from build123d import *

# Parameters (mm, degrees)
BOSS_EXTRUDE1_DEPTH = 4
FILLET1_R           = 1
SKETCH2_W           = 6.5
SKETCH2_H           = 21
SKETCH2_W_2         = 3
SKETCH2_H_2         = 16
BOSS_EXTRUDE2_DEPTH = 3
CUT_EXTRUDE3_DEPTH  = 94.63893421


with BuildPart() as part:
    # Sketch1 → Boss-Extrude1 (new body)
    with BuildSketch(Plane.XY):
        Polygon((0, 0), (52, 0), (52, 4), (90.5, 4), (90.5, 19), (52, 19), (52, 23), (0, 23), align=None)
    extrude(amount=BOSS_EXTRUDE1_DEPTH)

    # Fillet1
    fillet1_edges = [part.edges().sort_by_distance(p)[0] for p in [
        (0, 23, 2),
        (52, 23, 2),
        (52, 19, 2),
        (90.5, 19, 2),
        (90.5, 4, 2),
        (52, 4, 2),
        (52, 0, 2),
        (0, 0, 2),
    ]]
    fillet(fillet1_edges, radius=FILLET1_R)

    # Sketch2 → Boss-Extrude2 (add)
    with BuildSketch(Plane.XY.offset(4)):
        with Locations((46.75, 11.5)):
            Rectangle(SKETCH2_W, SKETCH2_H)
        with Locations((46.75, 11.5)):
            Rectangle(SKETCH2_W_2, SKETCH2_H_2, mode=Mode.SUBTRACT)
    extrude(amount=BOSS_EXTRUDE2_DEPTH)

    # Sketch3 → Cut-Extrude3 (cut, through all)
    with BuildSketch(Plane(origin=(0, 0, 0), x_dir=(-1, 0, 0), z_dir=(0, 0, -1))):
        with BuildLine():
            Line((-53.7, 14), (-52.3, 14))
            ThreePointArc((-52.3, 14), (-51.734314575, 14.234314575), (-51.5, 14.8))
            Line((-51.5, 14.8), (-51.5, 16.2))
            ThreePointArc((-51.5, 16.2), (-51.734314575, 16.765685425), (-52.3, 17))
            Line((-52.3, 17), (-53.7, 17))
            ThreePointArc((-53.7, 17), (-54.265685425, 16.765685425), (-54.5, 16.2))
            Line((-54.5, 16.2), (-54.5, 14.8))
            ThreePointArc((-54.5, 14.8), (-54.265685425, 14.234314575), (-53.7, 14))
        make_face()
        with BuildLine():
            Line((-52.3, 10), (-53.7, 10))
            ThreePointArc((-53.7, 10), (-54.265685425, 10.234314575), (-54.5, 10.8))
            Line((-54.5, 10.8), (-54.5, 12.2))
            ThreePointArc((-54.5, 12.2), (-54.265685425, 12.765685425), (-53.7, 13))
            Line((-53.7, 13), (-52.3, 13))
            ThreePointArc((-52.3, 13), (-51.734314575, 12.765685425), (-51.5, 12.2))
            Line((-51.5, 12.2), (-51.5, 10.8))
            ThreePointArc((-51.5, 10.8), (-51.734314575, 10.234314575), (-52.3, 10))
        make_face()
        with BuildLine():
            Line((-53.7, 6), (-52.3, 6))
            ThreePointArc((-52.3, 6), (-51.734314575, 6.234314575), (-51.5, 6.8))
            Line((-51.5, 6.8), (-51.5, 8.2))
            ThreePointArc((-51.5, 8.2), (-51.734314575, 8.765685425), (-52.3, 9))
            Line((-52.3, 9), (-53.7, 9))
            ThreePointArc((-53.7, 9), (-54.265685425, 8.765685425), (-54.5, 8.2))
            Line((-54.5, 8.2), (-54.5, 6.8))
            ThreePointArc((-54.5, 6.8), (-54.265685425, 6.234314575), (-53.7, 6))
        make_face()
    extrude(amount=-CUT_EXTRUDE3_DEPTH, mode=Mode.SUBTRACT)


solid = part.part
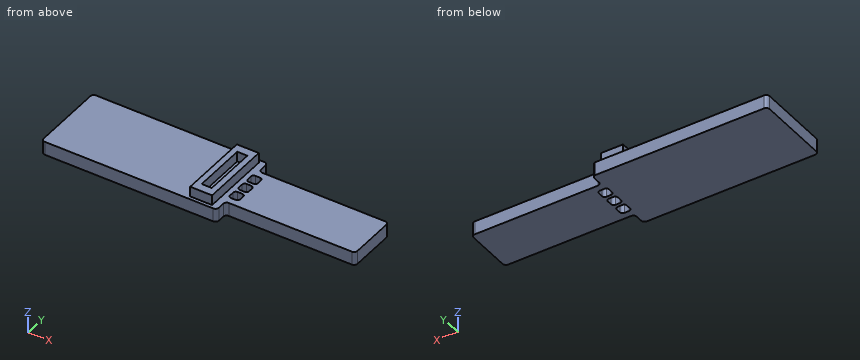
Could you check a few things on this model? Use its own coordinates, in mm. Give positions to 0.01 mm unless a question says otherwise; leave off trailing zeros. Order: outer loops, then holes, each group sorted by start corner. A loop starts at its lowest first (then second) coordinate and runs counter-clockwise, first axis right, second up. Notation, with made-up numbers: (44.5, 54) -> (70.5, 54) arc R14 ccw to (70.5, 69) -> close; hole circle Ø9 at (25.25, -13). An arc over 180 degrees is marked (long way). Answer in a Markdown table with one row per item. Add a question column.
Item 1: Imagine slicing it at C-C (x = 74.5). List the corners of the cut face in (y, z) for me.
Item 2: I'm going to push flat-ended pins straight in: P1, Ø0.7, axis at x = 53, z = 2.5, coming from the -Y side; P2, Ø0.9, axis at x = 47.5, z = 6, coming from the -Y side; P3, Ø11.5, axis at x = 61, y = 13.5, coming from the +Z side. Where does each tip first touch, or does it pass through?
Item 3: Imagine slicing it at A-A (z = 4.75). List the corners of the cut face in (x, y) for me, and give its area (3 significant figures).
Item 4: Imagine slicing it at D-D (x = 34.5). List the corners of the cut face in (y, z) for me.
Item 5: Imagine slicing it at B-B (y = 2.25). List the corners of the cut face in (x, z) for me, and give its area (4 significant figures).
Item 6: Please list where these lines run through material, in increasing order: probe 1 along X at (y, z) = (5.5, 4.5); probe 2 along X at (y, z) = (16, 1.75); probe 3 along Z at (x, y) = (42.5, 20.75).
Result:
| question | item | result |
|---|---|---|
| 1 | outline | (4, 0) -> (19, 0) -> (19, 4) -> (4, 4) -> close |
| 2 | P1 | y = 3.94 |
| 2 | P2 | y = 1 |
| 2 | P3 | z = 4 |
| 3 | outline | (43.5, 1) -> (50, 1) -> (50, 22) -> (43.5, 22) -> close; hole (45.25, 3.5) -> (48.25, 3.5) -> (48.25, 19.5) -> (45.25, 19.5) -> close |
| 3 | area | 88.5 mm2 |
| 4 | outline | (0, 0) -> (23, 0) -> (23, 4) -> (0, 4) -> close |
| 5 | outline | (0, 0) -> (52, 0) -> (52, 4) -> (50, 4) -> (50, 7) -> (43.5, 7) -> (43.5, 4) -> (0, 4) -> close |
| 5 | area | 227.5 mm2 |
| 6 | probe 1 | 43.5 to 45.25, 48.25 to 50 |
| 6 | probe 2 | 0 to 51.5, 54.5 to 90.5 |
| 6 | probe 3 | 0 to 4 |
